from build123d import *

# Parameters (mm, degrees)
SKETCH1_R           = 1.524
BOSS_EXTRUDE1_DEPTH = 2.54


with BuildPart() as part:
    # Sketch1 → Boss-Extrude1 (new body)
    with BuildSketch(Plane(origin=(0, 0, 0), x_dir=(0, 0, -1), z_dir=(1, 0, 0))):
        with BuildLine():
            Line((-50.098445601, 7.088580138), (-43.849100544, -8.683576435))
            Line((-43.849100544, -8.683576435), (4.658436215, -8.397602077))
            ThreePointArc((4.658436215, -8.397602077), (10.232240609, -7.180288327), (14.831146716, -3.804016594))
            Line((14.831146716, -3.804016594), (24.334060944, -3.804016594))
            ThreePointArc((24.334060944, -3.804016594), (28.629205553, 0.491128014), (24.334060944, 4.786272622))
            Line((24.334060944, 4.786272622), (14.134590219, 4.786272622))
            add(Edge.make_bspline(
                [(14.134590219, 4.786272622), (12.843386165, 4.731447756), (10.814047052, 3.6607913), (10.165897568, 0.480505822), (8.613444363, -0.857594594), (7.353623418, -1.210119508)],
                knots=[0, 0, 0, 0, 0.42442334, 0.587762542, 1, 1, 1, 1], degree=3))
            Line((7.353623418, -1.210119508), (-40.305133261, -1.491089915))
            Line((-40.305133261, -1.491089915), (-41.553433836, -0.257421693))
            Line((-41.553433836, -0.257421693), (-41.553433836, 2.122185781))
            Line((-41.553433836, 2.122185781), (-44.766052446, 2.122185781))
            Line((-44.766052446, 2.122185781), (-44.766052446, 5.877981651))
            Line((-44.766052446, 5.877981651), (-42.008654347, 5.877981651))
            Line((-42.008654347, 5.877981651), (-42.025194626, 8.683576435))
            Line((-42.025194626, 8.683576435), (-50.098445601, 8.683576435))
            Line((-50.098445601, 8.683576435), (-50.098445601, 7.088580138))
        make_face()
        with Locations((15.07250618, 0.779338165)):
            Circle(SKETCH1_R, mode=Mode.SUBTRACT)
    extrude(amount=BOSS_EXTRUDE1_DEPTH)


solid = part.part
Input: part model. Units: mm. Frame: model coordinates. A direction names the side the tool comes from. Give positions to 0.01 mm unless a question says otherwise; leave off trailing zeros. Write each loop counter-clockwise with the first axis right and the second up, starting at its lowest first coordinate (ties: lowest second). Pieces come first, ordered by that corner, then holes. Notation, with made-up numbers: (56.5, 11.5) -> (105.5, 11.5) arc R27 ccw to (105.5, 45.5) -> close; hole circle Ø1 at (-27.5, 3). An arc over 180 degrees is marked (long way). Use one line per item in the form item = value. Start each with the question number.
1) Set-up query: faces 4 (the flat face through (1, 5.878, 43)), 5 (the flat face through (1, 1, 41.553)), 6 (the flat face through (1, -3.804, -20)). Return all of +Z, -Z, +X, -X, +Y, -Y with unobstructed straight access to the full face (end or side cutting, diameter ignored); none if empty.
2) Draft query along Z for faces 1 (the cylindrical face through (1.252, -7.213, -10.159)), 2 (the flat face through (1.252, -0.883, 40.921)), 3 (the flat face through (1, 4.786, -19)). Return one class per face: pulls with the +Z half, pulls with the -Z half, needs draft (parallel to the pull), parting line crosses it, or undercut.
3) Ray query, probe 1 along Y at (x, z) = (0.75, 43.5); probe 2 along Y at (x, z) = (2.2, -17.5); probe 3 along Z at (x, y) = (0.4, 7.25). Return the intervals inside material, ascending. Write a range as from..to.
4) Pin query (flat end, axial travel): pin 1 (1.5 mm diameter, centred on x = 0.5, y = -3.5, fed in from -Z); pin 2 (0.8 mm diameter, centred on x = 1.5, y = 3, fed in from -Z); pin 3 (1.3 mm diameter, centred on x = 1.5, z = -17.5, fed in from -Y). Return the tip coordinate at first contact, or that it passes through.
5) Section query A-A on z = 14. Return the cut outline in (x, y).
6) Section query B-B on y = -7.25. Return the cut outline in (x, z), then the cut area to 3 significant figures.
Outcome:
q1.face_4 = -Z, +X, -X
q1.face_5 = +X, -X, +Y
q1.face_6 = -Z, +X, -X, -Y
q2.face_1 = pulls with the -Z half
q2.face_2 = undercut
q2.face_3 = needs draft
q3.probe_1 = -8.68..2.12, 5.88..8.68
q3.probe_2 = -3.8..4.79
q3.probe_3 = 42.02..50.1
q4.pin_1 = -27.15
q4.pin_2 = -28.08
q4.pin_3 = -3.8
q5.outline = (0, -8.51) -> (2.54, -8.51) -> (2.54, -1.34) -> (0, -1.34) -> close
q6.outline = (0, -10.08) -> (2.54, -10.08) -> (2.54, 44.42) -> (0, 44.42) -> close
q6.area = 138 mm^2
